```python
from build123d import *

# Parameters (mm, degrees)
SKETCH_4_W      = 15.6
SKETCH_4_H      = 15.6
EXTRUDE_1_DEPTH = 1.1
EXTRUDE_2_DEPTH = 4.9
SKETCH_7_W      = 13.9
SKETCH_7_H      = 13.6
EXTRUDE_4_DEPTH = 5
SKETCH_6_R      = 1.95
EXTRUDE_3_DEPTH = 3.3
SKETCH_8_W      = 1.2
SKETCH_8_H      = 4
SKETCH_8_W_2    = 4
SKETCH_8_H_2    = 1.2
EXTRUDE_5_DEPTH = 3.9
SKETCH_9_W      = 1
SKETCH_9_H      = 0.3
EXTRUDE_6_DEPTH = 3.8


with BuildPart() as part:
    # 草图4 → 凸台-拉伸1 (new body)
    with BuildSketch(Plane(origin=(0, 0, 0), x_dir=(1, 0, 0), z_dir=(0, 1, 0))):
        Rectangle(SKETCH_4_W, SKETCH_4_H)
    extrude(amount=EXTRUDE_1_DEPTH)

    # 草图5 → 凸台-拉伸2 (add, symmetric)
    with BuildSketch(Plane(origin=(0, 0, 0), x_dir=(0, 0, -1), z_dir=(1, 0, 0))):
        Polygon((-7.25, 1.1), (7.25, 1.1), (5.6, 6.3), (-3.4, 6.3), align=None)
    extrude(amount=EXTRUDE_2_DEPTH, both=True)

    # 草图7 → 凸台-拉伸4 (add)
    with BuildSketch(Plane.XZ):
        Rectangle(SKETCH_7_W, SKETCH_7_H)
    extrude(amount=EXTRUDE_4_DEPTH)

    # 草图6 → 凸台-拉伸3 (add)
    with BuildSketch(Plane.XZ.offset(5)):
        with Locations(Location((0, 0, 0), (0, 0, 270))):
            Circle(SKETCH_6_R)
    extrude(amount=EXTRUDE_3_DEPTH)

    # 草图8 → 凸台-拉伸5 (add)
    with BuildSketch(Plane(origin=(0, 6.3, 0), x_dir=(1, 0, 0), z_dir=(0, 1, 0))):
        Rectangle(SKETCH_8_W, SKETCH_8_H)
        Rectangle(SKETCH_8_W_2, SKETCH_8_H_2)
    extrude(amount=EXTRUDE_5_DEPTH)

    # 草图9 → 凸台-拉伸6 (add)
    with BuildSketch(Plane.XZ.offset(5)):
        with Locations((2.54, -5.01)):
            Rectangle(SKETCH_9_W, SKETCH_9_H)
        with Locations((-3.81, -2.54)):
            Rectangle(SKETCH_9_W, SKETCH_9_H)
    extrude(amount=EXTRUDE_6_DEPTH)


solid = part.part
```
Work out the finished part from the listing and answer in its coordinate system (mm). A direction names the side the tool comes from. Coordinates: 2 decimals unless noted, no trailing zeros. Write each loop counter-clockwise with the first axis right and the second up, starting at its lowest first coordinate (ties: lowest second). Pieces come first, ordered by that corner, then holes.
Q1. Each of these flat-tipped pins is pushed along its axis until it touches: pin 1 Ø1.1 at (x, y) = (-3.5, -7.5) entering from -Z; pin 2 Ø1.5 at (y, z) = (9, 1) entering from -X; pin 3 Ø8 at (x, y) = (-6, 7) entering from -Z. Where does it stop, or does it pass through?
Q2. A cutting plane is placed at D-D, the plane y = 7.75. Give the vertices of the cut face in (x, z).
Q3. Find the intervals of material crossed by line 1 (Y direction, x = -2.5, z = -1.75); line 2 (Z direction, x = 2.75, y = -2.75); line 3 (Z direction, x = -0.25, y = 8.25), in increasing order.
Q4. A cutting plane is placed at B-B, the plane x = 4. Give the vertices of the cut face in (y, z).
Q5. Which of the six approach directions +Z, -Z, +X, -X, +Y, -Y give full straight-line access (tool end or side, diameter ignored) to faces 1 (the face through (-4.9, 4, 0)), 2 (the face through (-1.187, -6.627, 1.547)), 3 (the face through (6.95, -2, 0))?
Q6. A cutting plane is placed at A-A, the plane y = -6.5. Give the vertices of the cut face in (x, z), then the cut area to 3 significant figures.
Q7. A cutting plane is placed at C-C, the plane z = 0. Give the vertices of the cut face in (x, y), then the cut area to 3 significant figures.
Findings below:
1. pin 1: stops at z = -2.69
1. pin 2: stops at x = -2
1. pin 3: stops at z = -6.6
2. outline: (-2, -0.6) - (-0.6, -0.6) - (-0.6, -2) - (0.6, -2) - (0.6, -0.6) - (2, -0.6) - (2, 0.6) - (0.6, 0.6) - (0.6, 2) - (-0.6, 2) - (-0.6, 0.6) - (-2, 0.6) - close
3. line 1: y = -5 to 6.3
3. line 2: z = -6.8 to 6.8
3. line 3: z = -2 to 2
4. outline: (-5, -6.8) - (0, -6.8) - (0, -7.8) - (1.1, -7.8) - (1.1, -7.25) - (6.3, -5.6) - (6.3, 3.4) - (1.1, 7.25) - (1.1, 7.8) - (0, 7.8) - (0, 6.8) - (-5, 6.8) - close
5. face 1: +Z, -Z, -X, +Y
5. face 2: -Y
5. face 3: +Z, -Z, +X, -Y
6. outline: (-4.31, -2.69) - (-3.31, -2.69) - (-3.31, -2.39) - (-4.31, -2.39) - close; circle Ø3.9 at (0, 0); (2.04, -5.16) - (3.04, -5.16) - (3.04, -4.86) - (2.04, -4.86) - close
6. area: 12.5 mm2
7. outline: (-7.8, 0) - (-6.95, 0) - (-6.95, -5) - (-1.95, -5) - (-1.95, -8.3) - (1.95, -8.3) - (1.95, -5) - (6.95, -5) - (6.95, 0) - (7.8, 0) - (7.8, 1.1) - (4.9, 1.1) - (4.9, 6.3) - (2, 6.3) - (2, 10.2) - (-2, 10.2) - (-2, 6.3) - (-4.9, 6.3) - (-4.9, 1.1) - (-7.8, 1.1) - close
7. area: 166 mm2
